Here's how the part is built. I have some questions about the finished solid (model axes, mm). Coordinates: 2 decimals unless noted, no trailing zeros. Loops run counter-clockwise (first coordinate to the right, second up) from the corner with the lowest first, then second, coordinate; pieces in that order, holes last.
Autodesk Inventor part; units mm, degrees
ref_plane "YZ Plane" through (0, 0, 0) normal (1, 0, 0) x (0, 1, 0)
ref_plane "XZ Plane" through (0, 0, 0) normal (0, 1, 0) x (-1, 0, 0)
ref_plane "XY Plane" through (0, 0, 0) normal (0, 0, 1) x (1, 0, 0)
sketch "Sketch1" plane through (0, 0, 0) normal (0, 0, 1) x (1, 0, 0)
  circle A0 centre (0, 0) radius 34
  dimension "d0" = 68
extrude "Extrusion1" add sketch "Sketch1" against normal blind 2.54
sketch "Sketch2" plane through (0, 0, -2.54) normal (0, 0, -1) x (-1, 0, 0)
  line L0 (5, 5) -> (-5, 5)
  line L1 (-5, 5) -> (-5, -5)
  line L2 (-5, -5) -> (5, -5)
  line L3 (5, -5) -> (5, 5)
  line L4 (5, 5) -> (-5, -5) construction
  line L5 (-5, 5) -> (5, -5) construction
  point P0 (0, 0)
  dimension "d3" = 10
extrude "Extrusion2" cut sketch "Sketch2" against normal through all
sketch "Sketch3" plane through (0, 0, -2.54) normal (0, 0, -1) x (-1, 0, 0)
  circle A0 centre (0, 0) radius 26 construction
  line L0 (3, -24) -> (-3, -24)
  line L1 (-3, -24) -> (-3, -28)
  line L2 (-3, -28) -> (3, -28)
  line L3 (3, -28) -> (3, -24)
  line L4 (3, -24) -> (-3, -28) construction
  line L5 (-3, -24) -> (3, -28) construction
  line L6 (8.648, -26.7995) -> (14.1293, -24.3591)
  line L7 (14.1293, -24.3591) -> (12.5023, -20.7049)
  line L8 (7.021, -23.1453) -> (8.648, -26.7995)
  line L9 (12.5023, -20.7049) -> (7.021, -23.1453)
  line L10 (18.8007, -20.9651) -> (22.8154, -16.5062)
  line L11 (22.8154, -16.5062) -> (19.8429, -13.8297)
  line L12 (15.8281, -18.2886) -> (18.8007, -20.9651)
  line L13 (19.8429, -13.8297) -> (15.8281, -18.2886)
  line L14 (25.7025, -11.5056) -> (27.5566, -5.7993)
  line L15 (27.5566, -5.7993) -> (23.7524, -4.5632)
  line L16 (21.8983, -10.2696) -> (25.7025, -11.5056)
  line L17 (23.7524, -4.5632) -> (21.8983, -10.2696)
  line L18 (28.1602, -0.0568) -> (27.533, 5.9104)
  line L19 (27.533, 5.9104) -> (23.5549, 5.4922)
  line L20 (24.1821, -0.4749) -> (28.1602, -0.0568)
  line L21 (23.5549, 5.4922) -> (24.1821, -0.4749)
  line L22 (25.7487, 11.4019) -> (22.7487, 16.5981)
  line L23 (22.7487, 16.5981) -> (19.2846, 14.5981)
  line L24 (22.2846, 9.4019) -> (25.7487, 11.4019)
  line L25 (19.2846, 14.5981) -> (22.2846, 9.4019)
  line L26 (18.885, 20.8891) -> (14.0309, 24.4158)
  line L27 (14.0309, 24.4158) -> (11.6798, 21.1798)
  line L28 (16.5339, 17.6531) -> (18.885, 20.8891)
  line L29 (11.6798, 21.1798) -> (16.5339, 17.6531)
  line L30 (8.756, 26.7644) -> (2.8871, 28.0119)
  line L31 (2.8871, 28.0119) -> (2.0554, 24.0993)
  line L32 (7.9243, 22.8518) -> (8.756, 26.7644)
  line L33 (2.0554, 24.0993) -> (7.9243, 22.8518)
  line L34 (-2.8871, 28.0119) -> (-8.756, 26.7644)
  line L35 (-8.756, 26.7644) -> (-7.9243, 22.8518)
  line L36 (-2.0554, 24.0993) -> (-2.8871, 28.0119)
  line L37 (-7.9243, 22.8518) -> (-2.0554, 24.0993)
  line L38 (-14.0309, 24.4158) -> (-18.885, 20.8891)
  line L39 (-18.885, 20.8891) -> (-16.5339, 17.6531)
  line L40 (-11.6798, 21.1798) -> (-14.0309, 24.4158)
  line L41 (-16.5339, 17.6531) -> (-11.6798, 21.1798)
  line L42 (-22.7487, 16.5981) -> (-25.7487, 11.4019)
  line L43 (-25.7487, 11.4019) -> (-22.2846, 9.4019)
  line L44 (-19.2846, 14.5981) -> (-22.7487, 16.5981)
  line L45 (-22.2846, 9.4019) -> (-19.2846, 14.5981)
  line L46 (-27.533, 5.9104) -> (-28.1602, -0.0568)
  line L47 (-28.1602, -0.0568) -> (-24.1821, -0.4749)
  line L48 (-23.5549, 5.4922) -> (-27.533, 5.9104)
  line L49 (-24.1821, -0.4749) -> (-23.5549, 5.4922)
  line L50 (-27.5566, -5.7993) -> (-25.7025, -11.5056)
  line L51 (-25.7025, -11.5056) -> (-21.8983, -10.2696)
  line L52 (-23.7524, -4.5632) -> (-27.5566, -5.7993)
  line L53 (-21.8983, -10.2696) -> (-23.7524, -4.5632)
  line L54 (-22.8154, -16.5062) -> (-18.8007, -20.9651)
  line L55 (-18.8007, -20.9651) -> (-15.8281, -18.2886)
  line L56 (-19.8429, -13.8297) -> (-22.8154, -16.5062)
  line L57 (-15.8281, -18.2886) -> (-19.8429, -13.8297)
  line L58 (-14.1293, -24.3591) -> (-8.648, -26.7995)
  line L59 (-8.648, -26.7995) -> (-7.021, -23.1453)
  line L60 (-12.5023, -20.7049) -> (-14.1293, -24.3591)
  line L61 (-7.021, -23.1453) -> (-12.5023, -20.7049)
  point P0 (0, -26)
  dimension "d6" = 52
  dimension "d7" = 4
  dimension "d8" = 6
  dimension "d11" = 360
extrude "Extrusion3" cut sketch "Sketch3" against normal through all
sketch "Sketch4" plane through (0, 0, 0) normal (0, 0, 1) x (1, 0, 0)
  line L0 (-18.7521, 0) -> (0, 0) construction
  line L1 (0, 0) -> (0, 18.7521) construction
  circle A0 centre (0, 0) radius 18.7521 construction
  point P0 (-16.2398, -9.376)
  point P1 (16.2398, -9.3761)
  dimension "d15" = 37.5042
  dimension "d16" = 18.7521
  dimension "d17" = 90
  dimension "d20" = 360
hole "Hole1" at (0, 18.7521, 0) at (-16.2398, -9.376, 0) at (16.2398, -9.3761, 0) direction (0, 0, -1) diameter 4.318 end through all
equation "\"d1\" = CoverDepth"
equation "\"d6\" = 2 * LightRingCenterRadius"
equation "\"d15\" = SupportScrewsDiameter"
equation "\"d16\" = 0.5 * SupportScrewsDiameter"
properties part number "MountCover" material "Polycarbonate, Clear"
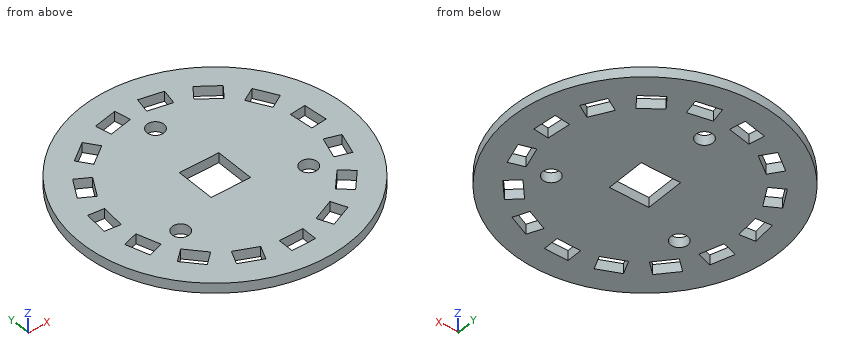
Q1. Suppose I cut it at D-D on z = -1.15. State how many separate pieces and enclosed holes the cut face has, and give its area (3 significant figures).
Q2. Suppose I cut it at C-C on y = -15. Write out the boundary of the cut face in (x, z).
Q3. Suppose I cut it at A-A on x = 0. Write out the boundary of the cut face in (y, z), and give its area (3 significant figures).
Q4. Please list where these lines run through material, in increasing order: probe 1 along X at (y, z) = (21, -0.45); probe 2 along Y at (x, z) = (-24.5, -0.35); probe 3 along X at (y, z) = (13.5, -0.05).
Q5. Will these pins go through, and if not, where does the flat tip stop? P1, Ø1.3, axis at x = -2, z = -1, coming from the +Y side; P2, Ø1.3, axis at y = 2.5, z = -1, coming from the -X side; P3, Ø1.3, axis at y = -25.5, z = -2, coming from the -X side.
Q6. Suppose I cut it at B-B on y = 13. Write out the boundary of the cut face in (x, z).
Check values:
1. separate pieces: 1
1. enclosed holes: 19
1. area: 3,130 mm2
2. outline: (-30.51, -2.54) - (-21.14, -2.54) - (-21.14, 0) - (-30.51, 0) - close; (-18.79, -2.54) - (18.79, -2.54) - (18.79, 0) - (-18.79, 0) - close; (21.14, -2.54) - (30.51, -2.54) - (30.51, 0) - (21.14, 0) - close
3. outline: (-34, -2.54) - (-28, -2.54) - (-28, 0) - (-34, 0) - close; (-24, -2.54) - (-5, -2.54) - (-5, 0) - (-24, 0) - close; (5, -2.54) - (16.59, -2.54) - (16.59, 0) - (5, 0) - close; (20.91, -2.54) - (34, -2.54) - (34, 0) - (20.91, 0) - close
3. area: 126 mm2
4. probe 1: x = -26.74 to -18.73, -11.93 to 11.93, 18.73 to 26.74
4. probe 2: y = -23.57 to -11.11, -4.81 to -0.44, 5.59 to 10.68, 13.56 to 23.57
4. probe 3: x = -31.2 to -24.54, -19.92 to 19.92, 24.54 to 31.2
5. P1: stops at y = 33.97
5. P2: stops at x = -33.95
5. P3: stops at x = -23.21
6. outline: (-31.42, -2.54) - (-24.83, -2.54) - (-24.83, 0) - (-31.42, 0) - close; (-20.21, -2.54) - (20.21, -2.54) - (20.21, 0) - (-20.21, 0) - close; (24.83, -2.54) - (31.42, -2.54) - (31.42, 0) - (24.83, 0) - close
